```python
from build123d import *

# Parameters (mm, degrees)
BOSS_EXTRUDE1_DEPTH = 6.35
BOSS_EXTRUDE3_DEPTH = 25
SKETCH3_W           = 203.2
SKETCH3_H           = 6.35
CUT_EXTRUDE1_DEPTH  = 10


with BuildPart() as part:
    # Sketch1 → Boss-Extrude1 (new body)
    with BuildSketch(Plane.XY):
        Polygon((0, 0), (203.2, 0), (303.2, 50), (203.2, 100), (0, 100), (-100, 50), align=None)
    extrude(amount=BOSS_EXTRUDE1_DEPTH)

    # Sketch2 → Boss-Extrude3 (add)
    with BuildSketch(Plane(origin=(0, 0, 0), x_dir=(-1, 0, 0), z_dir=(0, 0, -1))):
        Polygon((-177.8, 12.7), (-203.2, 12.7), (-203.2, 19.05), (-177.8, 19.05), (-177.8, 25.05), (-209.2, 25.05), (-209.2, 6.7), (-177.8, 6.7), align=None)
        Polygon((6, 6.7), (6, 25.05), (-25.4, 25.05), (-25.4, 19.05), (0, 19.05), (0, 12.7), (-25.4, 12.7), (-25.4, 6.7), align=None)
    extrude(amount=BOSS_EXTRUDE3_DEPTH)

    # Sketch3 → Cut-Extrude1 (cut)
    with BuildSketch(Plane(origin=(0, 0, 0), x_dir=(-1, 0, 0), z_dir=(0, 0, -1))):
        with Locations((-101.6, 15.875)):
            Rectangle(SKETCH3_W, SKETCH3_H)
    extrude(amount=-CUT_EXTRUDE1_DEPTH, mode=Mode.SUBTRACT)


solid = part.part
```
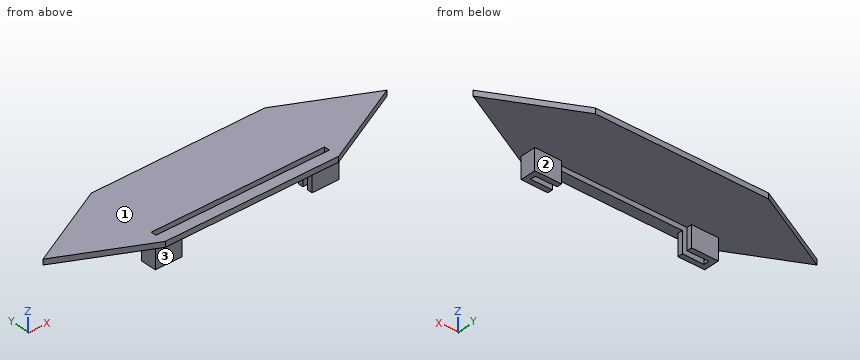
Part model, mm, in its own coordinate system. Face numbers are marked on the shaded views. A direction names the side the tool comes from. Round coordinates to 2 decimals unless told otherwise and drop trailing zeros. Write each loop counter-clockwise with the first axis right and the second up, starting at its lowest first coordinate (ties: lowest second). Pieces come first, ordered by that corner, then holes. Notation, with made-up numbers: M -1.5,76.5 L 4.5,76.5 A8 cw 4.5,83.5 Z; hole C -5.75,-8.5 d8. An arc over 180 degrees is marked long. Answer as CSV lines item,"result". Start each with the question number.
1) Band-saw the part on A-A (x = 22). List the corners of the cut face in (y, z).
2) Band-saw the part on C-C (y = 83). List the corners of the cut face in (x, z), then the cut area to 3 significant figures.
3) Band-saw the part on B-B (z = -19). List the corners of the cut face in (x, y).
4) Which spindle directions (+Z, -Z, +X, -X, +Y, -Y) get a long thin tool onto all of the face, cutting with end or side? Do the marked faces 1, 2 and 3. Say none if no direction does.
5) Band-saw the part on D-D (x = 133.5). List the corners of the cut face in (y, z), then the cut area to 3 significant figures.
6) Drill centre lines: L1, parallel to Y at x = 185.5, z = -15.5; L2, parallel to X at y = 15.5, z = -22.5; L3, parallel to Z at x = -77, y = 61. Where is each one in solid material? Low to high.
7) Drop flat-ended pins along their axis: pin 1 (7.5 mm diameter, centred on x = 10, z = -11.5, fed in from +Y); pin 2 (5 mm diameter, centred on x = 134, y = 62, fed in from -Z); pin 3 (1.9 mm diameter, centred on y = 15, z = -17, fed in from -X); pin 4 (15.5 mm diameter, centred on x = 120, z = -8.5, fed in from +Y). Give the stop position or say it passes through.
Worked out:
1,outline,"M 0,0 L 6.7,0 L 6.7,-25 L 12.7,-25 L 12.7,6.35 L 0,6.35 Z; M 19.05,-25 L 25.05,-25 L 25.05,0 L 100,0 L 100,6.35 L 19.05,6.35 Z"
2,outline,"M -34,0 L 237.2,0 L 237.2,6.35 L -34,6.35 Z"
2,area,"1,720 mm²"
3,outline,"M -6,6.7 L 25.4,6.7 L 25.4,12.7 L 0,12.7 L 0,19.05 L 25.4,19.05 L 25.4,25.05 L -6,25.05 Z; M 177.8,6.7 L 209.2,6.7 L 209.2,25.05 L 177.8,25.05 L 177.8,19.05 L 203.2,19.05 L 203.2,12.7 L 177.8,12.7 Z"
4,face 1,"+Z, +X, -X, +Y, -Y"
4,face 2,"-Z, +X, -X, +Y"
4,face 3,"-Z, +X, -X, -Y"
5,outline,"M 0,0 L 12.7,0 L 12.7,6.35 L 0,6.35 Z; M 19.05,0 L 100,0 L 100,6.35 L 19.05,6.35 Z"
5,area,"595 mm²"
6,L1,"6.7 to 12.7, 19.05 to 25.05"
6,L2,"-6 to 0, 203.2 to 209.2"
6,L3,"0 to 6.35"
7,pin 1,"y = 25.05"
7,pin 2,"z = 0"
7,pin 3,"x = -6"
7,pin 4,"through"
